Input: dimensioned drawing with shaded views. Units: mm. Origin: part minimum x, y, z. A direction names the side the tool comes from. Round coordinates to 2 decimals unless told otherwise and drop trailing zeros. Order: outer loops, then holes, each group sorted by start corner. A loop starts at its lowest first (then second) coordinate and runs counter-clockwise, first axis right, second up. Notation, with made-up numbers: M 34,-18.75 L 93,-18.75 A33 ccw 93,15.25 Z; hole C -31,8.5 d2. An arc over 180 degrees is marked long. Put each result on its own line as item: value. Start each with the question number.
1) Draft query along X for the marked faces 1, 2 and 3. Return one class per face: pulls with the +X half, pulls with the -X half, needs draft (parallel to the pull), parting line crosses it, or undercut.
2) Section C-C, the plane y = 15.75. Return loops of the section in (x, z), then the cut area to 3 significant figures.
3) First-contact query: P1, Ø4.5, axis at x = 9.5, z = 4, coming from the -Y side; P2, Ø1, axis at x = 5, z = 1.5, coming from the -Y side; P3, Ø3, axis at x = 14, y = 3, coming from the +Z side. Flat tips, straight axial feed; report the tip coordinate or a pass-through.
4) Material intervals for probe 1 along X at (y, z) = (15.25, 9.25); probe 2 along Z at (x, y) = (10, 3); probe 3 along Y at (x, z) = (3.25, 5), sorted ascending. Write a range as [from, to].
5) Section B-B, the plane z = 5. Return loops of the section in (x, y), then the cut area to 3 significant figures.
6) Access query for the marked faces 4, 5 and 6. Directions: +Z, -Z, +X, -X, +Y, -Y. A direction counts if a zero-diameter tool reaches every point of the face in a straight line with its end or side. Return the directions, or none.
7) Section D-D, the plane x = 10. Return loops of the section in (y, z).
8) Section A-A, the plane x = 4.25. Return loops of the section in (y, z), then the cut area to 3 significant figures.
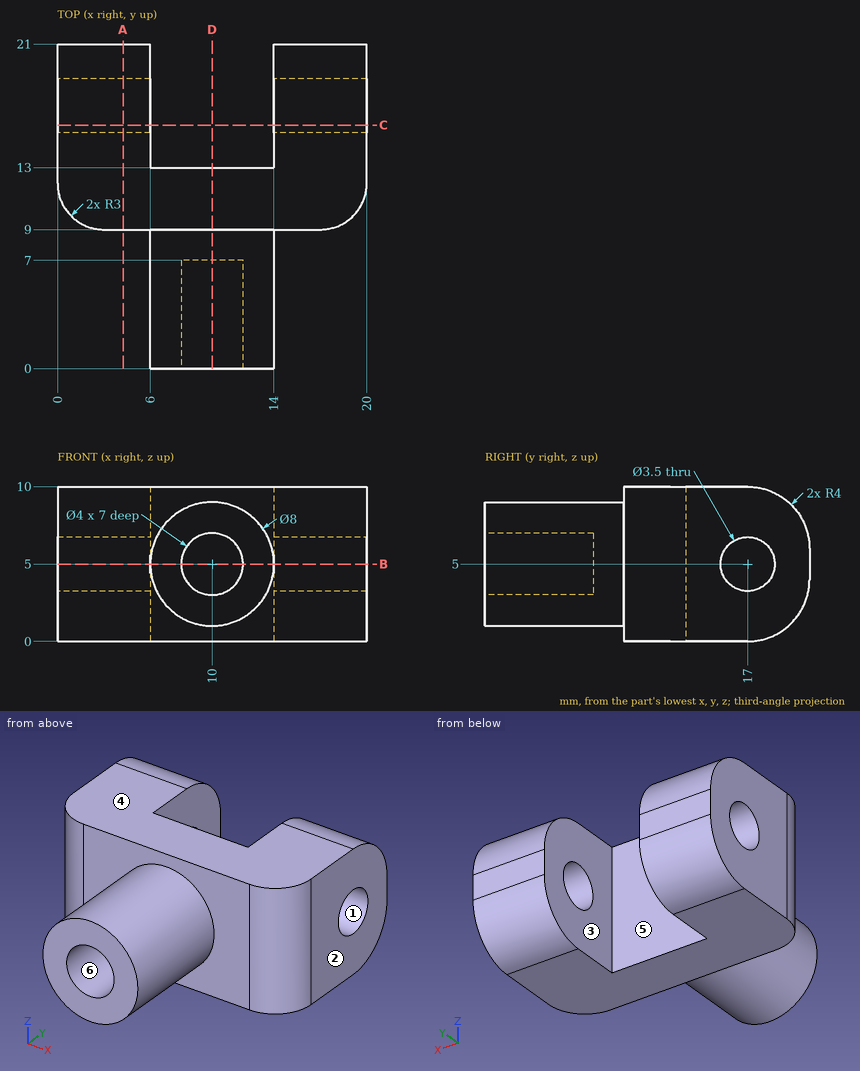
Result sheet:
1. face 1: needs draft
1. face 2: pulls with the +X half
1. face 3: undercut
2. outline: M 0,0 L 6,0 L 6,3.78 L 0,3.78 Z; M 0,6.22 L 6,6.22 L 6,10 L 0,10 Z; M 14,0 L 20,0 L 20,3.78 L 14,3.78 Z; M 14,6.22 L 20,6.22 L 20,10 L 14,10 Z
2. area: 90.6 mm2
3. P1: stops at y = 0
3. P2: stops at y = 9
3. P3: stops at z = 8.12
4. probe 1: x = [0, 6], [14, 20]
4. probe 2: z = [1, 3], [7, 9]
4. probe 3: y = [9, 15.25], [18.75, 21]
5. outline: M 0,12 A3 ccw 3,9 L 6,9 L 6,0 L 8,0 L 8,7 L 12,7 L 12,0 L 14,0 L 14,9 L 17,9 A3 ccw 20,12 L 20,15.25 L 14,15.25 L 14,13 L 6,13 L 6,15.25 L 0,15.25 Z; M 0,18.75 L 6,18.75 L 6,21 L 0,21 Z; M 14,18.75 L 20,18.75 L 20,21 L 14,21 Z
5. area: 174 mm2
6. face 4: +Z, +X, -X, +Y, -Y
6. face 5: +Z, -Z, +Y
6. face 6: -Y
7. outline: M 0,1 L 9,1 L 9,0 L 13,0 L 13,10 L 9,10 L 9,9 L 0,9 L 0,7 L 7,7 L 7,3 L 0,3 Z
8. outline: M 9,0 L 17,0 A4 ccw 21,4 L 21,6 A4 ccw 17,10 L 9,10 Z; hole C 17,5 d3.5
8. area: 104 mm2
